from build123d import *

# Parameters (mm, degrees)
SKETCH1_W           = 30
SKETCH1_H           = 30
BOSS_EXTRUDE1_DEPTH = 300
SKETCH2_W           = 100
SKETCH2_H           = 100
BOSS_EXTRUDE2_DEPTH = 5
CUT_EXTRUDE1_REACH  = 32
SKETCH3_R           = 2.5


with BuildPart() as part:
    # Sketch1 → Boss-Extrude1 (new body)
    with BuildSketch(Plane.XY):
        Rectangle(SKETCH1_W, SKETCH1_H)
    extrude(amount=BOSS_EXTRUDE1_DEPTH)

    # Sketch2 → Boss-Extrude2 (add)
    with BuildSketch(Plane(origin=(0, 15, 0), x_dir=(1, 0, 0), z_dir=(0, 1, 0))):
        with Locations((0, 50)):
            Rectangle(SKETCH2_W, SKETCH2_H)
    extrude(amount=-BOSS_EXTRUDE2_DEPTH)

    # Sketch3 → Cut-Extrude1 (cut, up to next)
    with BuildSketch(Plane(origin=(0, 15, 0), x_dir=(1, 0, 0), z_dir=(0, 1, 0)), mode=Mode.PRIVATE) as cut_extrude1_sk1:
        with Locations((-35, 15)):
            Circle(SKETCH3_R)
    cut_extrude1_tool1 = extrude(cut_extrude1_sk1.sketch, amount=-CUT_EXTRUDE1_REACH, mode=Mode.PRIVATE) & part.part
    add(cut_extrude1_tool1.solids().sort_by_distance((-35, 15, -15))[0], mode=Mode.SUBTRACT)
    # Sketch3 → Cut-Extrude1 (cut, up to next)
    with BuildSketch(Plane(origin=(0, 15, 0), x_dir=(1, 0, 0), z_dir=(0, 1, 0)), mode=Mode.PRIVATE) as cut_extrude1_sk2:
        with Locations((35, 15)):
            Circle(SKETCH3_R)
    cut_extrude1_tool2 = extrude(cut_extrude1_sk2.sketch, amount=-CUT_EXTRUDE1_REACH, mode=Mode.PRIVATE) & part.part
    add(cut_extrude1_tool2.solids().sort_by_distance((35, 15, -15))[0], mode=Mode.SUBTRACT)
    # Sketch3 → Cut-Extrude1 (cut, up to next)
    with BuildSketch(Plane(origin=(0, 15, 0), x_dir=(1, 0, 0), z_dir=(0, 1, 0)), mode=Mode.PRIVATE) as cut_extrude1_sk3:
        with Locations((-35, 85)):
            Circle(SKETCH3_R)
    cut_extrude1_tool3 = extrude(cut_extrude1_sk3.sketch, amount=-CUT_EXTRUDE1_REACH, mode=Mode.PRIVATE) & part.part
    add(cut_extrude1_tool3.solids().sort_by_distance((-35, 15, -85))[0], mode=Mode.SUBTRACT)
    # Sketch3 → Cut-Extrude1 (cut, up to next)
    with BuildSketch(Plane(origin=(0, 15, 0), x_dir=(1, 0, 0), z_dir=(0, 1, 0)), mode=Mode.PRIVATE) as cut_extrude1_sk4:
        with Locations((35, 85)):
            Circle(SKETCH3_R)
    cut_extrude1_tool4 = extrude(cut_extrude1_sk4.sketch, amount=-CUT_EXTRUDE1_REACH, mode=Mode.PRIVATE) & part.part
    add(cut_extrude1_tool4.solids().sort_by_distance((35, 15, -85))[0], mode=Mode.SUBTRACT)


solid = part.part
Design review of the part built by this model. Coordinates are the model's own, in mm. A direction names the side the tool comes from. Round coordinates to 2 decimals unless told otherwise and drop trailing zeros. Loops run counter-clockwise (first coordinate to the right, second up) from the corner with the lowest first, then second, coordinate; pieces in that order, holes last. Notation, with made-up numbers: (-23, 67) - (-14, 67) arc R21 ccw to (-14, 102) - close; hole circle Ø7 at (12.5, 30.25). An arc over 180 degrees is marked (long way). One line per item, written item: value. Start each with the question number.
1) To check wall thickness, follow L1, parallel to X at y = 13.7, z = -15; L2, parallel to Z at x = 35, y = 12.2; L3, parallel to X at y = 13, z = 212. State the ranges of each line that lie inside material, in increasing order. Write a range as from..to.
2) Consider section C-C on x = -6.5. Give the boundary of the cut face in (y, z), then the cut area to 3 significant figures.
3) Insertion check: pin 1 Ø8 at (x, z) = (-35, -15) entering from -Y; pin 2 Ø5.5 at (x, y) = (-40, 13) entering from +Z; pin 3 Ø1.5 at (y, z) = (4, 248) entering from +X. Each pin has a flat end and moves straight along its axis. Give the tip position at first contact, or say it passes through.
4) Consider section B-B on y = -8. Give the boundary of the cut face in (x, z).
5) Consider section A-A on x = 20. Give the boundary of the cut face in (y, z), then the cut area to 3 significant figures.
6) For faces 1 (the flat face through (0, -2, 0)), 2 (the flat face through (0, 0, 300)), list the 3-axis set-ups (+Z, -Z, +X, -X, +Y, -Y) from which the entire face can be reached by the end or side of a thin tool; tool diameter is ignored.
Reported:
1. L1: x = -50..-37.5, -32.5..32.5, 37.5..50
1. L2: z = -100..-87.5, -82.5..-17.5, -12.5..0
1. L3: x = -15..15
2. outline: (-15, 0) - (10, 0) - (10, -100) - (15, -100) - (15, 300) - (-15, 300) - close
2. area: 9,500 mm^2
3. pin 1: stops at y = 10
3. pin 2: stops at z = 0
3. pin 3: stops at x = 15
4. outline: (-15, 0) - (15, 0) - (15, 300) - (-15, 300) - close
5. outline: (10, -100) - (15, -100) - (15, 0) - (10, 0) - close
5. area: 500 mm^2
6. face 1: -Z, +X, -X, -Y
6. face 2: +Z, +X, -X, +Y, -Y
